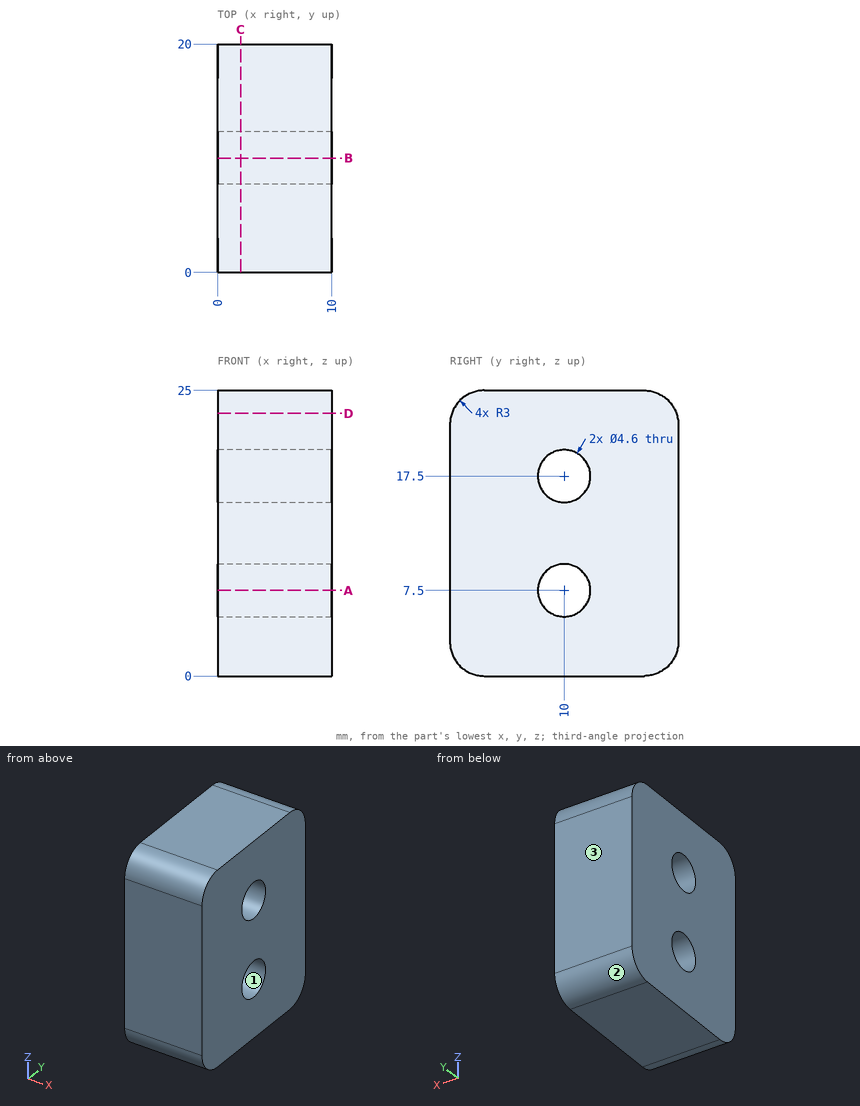
Geometry: see drawing. Coordinates: mm, zero at the bounding-box minimum. Give positions to 0.01 mm unless a question says otherwise; leave off trailing zeros. Order: outer loops, then holes, each group sorted by start corner. A loop starts at its lowest first (then second) coordinate and runs counter-clockwise, first axis right, second up. Notation, with made-up numbers: (33.5, 24.25) -> (54.5, 24.25) arc R22 cw to (54.5, 46.25) -> close; hole circle Ø8 at (-8, -26.5). An arc over 180 degrees is marked (long way). Write each question's results on one line, items separated by ' | '. Start each with the question number.
1) Section A-A (z = 7.5). Return loops of the section in (x, y), then the cut area to 3 significant figures.
2) Draft query along Z for the marked faces 1, 2 and 3. Return one class per face: pulls with the +Z half, pulls with the -Z half, needs draft (parallel to the pull), parting line crosses it, or undercut.
3) Section B-B (y = 10). Return loops of the section in (x, z).
4) Section C-C (x = 2). Return loops of the section in (y, z).
5) Section D-D (z = 23). Return loops of the section in (x, y), then the cut area to 3 significant figures.
6) Line query: line 1 (Y direction, x = 3.5, z = 7.5); line 2 (Y direction, x = 6, z = 19.5). Output: solid intervals per line, ascending. Write a range as from..to.
Calculated:
1) outline: (0, 0) -> (10, 0) -> (10, 7.7) -> (0, 7.7) -> close; (0, 12.3) -> (10, 12.3) -> (10, 20) -> (0, 20) -> close | area: 154 mm2
2) face 1: undercut | face 2: pulls with the -Z half | face 3: needs draft
3) outline: (0, 0) -> (10, 0) -> (10, 5.2) -> (0, 5.2) -> close; (0, 9.8) -> (10, 9.8) -> (10, 15.2) -> (0, 15.2) -> close; (0, 19.8) -> (10, 19.8) -> (10, 25) -> (0, 25) -> close
4) outline: (0, 3) arc R3 ccw to (3, 0) -> (17, 0) arc R3 ccw to (20, 3) -> (20, 22) arc R3 ccw to (17, 25) -> (3, 25) arc R3 ccw to (0, 22) -> close; hole circle Ø4.6 at (10, 7.5); hole circle Ø4.6 at (10, 17.5)
5) outline: (0, 0.17) -> (10, 0.17) -> (10, 19.83) -> (0, 19.83) -> close | area: 197 mm2
6) line 1: 0..7.7, 12.3..20 | line 2: 0..8.86, 11.14..20
